Input: part model. Units: mm. Frame: model coordinates. Give positions to 0.01 mm unless a question says otherwise; leave off trailing zeros. Use CSV: the item, a comma, the result in double quotes. Start each with the question number.
Q1. Material intervals for line 1 along Z through (x, y) = (152, 2.9); line 2 along X through (y, z) = (3, -79.5); line 3 along X through (y, z) = (4.55, -16), sorted ascending.
Q2. Pin query (flat end, axial travel): pin 1 (1.5 mm diameter, centred on y = 2.5, z = -39, fed in from -X); pin 2 (2.5 mm diameter, centred on x = 96, z = -79.5, fed in from -Y); pin 3 (2 mm diameter, centred on y = 0.5, z = 15, fed in from +X); pin 4 (2 mm diameter, centred on x = 5, y = 3, fed in from -Z). Return the tip coordinate at first contact, or that it passes through.
Q3. Section A-A, the plane y = 3.25. State how many separate pieces and enclosed holes the cut face has, plus the area to 3 significant figures.
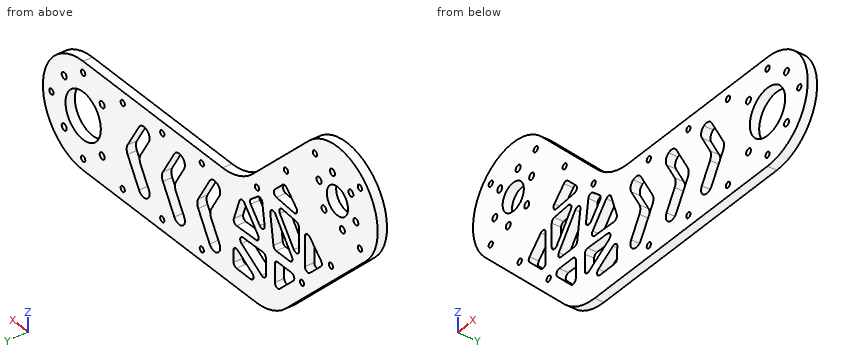
from build123d import *

# Parameters (mm, degrees)
SKETCH_1_R          = 28.5
EXTRUDE_1_DEPTH     = 5
FILLET_1_R          = 30
FILLET_2_R          = 30
CUT_EXTRUDE_1_DEPTH = 17
FILLET_3_R          = 5
FILLET_4_R          = 4
SKETCH_3_R          = 1.75
CUT_EXTRUDE_2_DEPTH = 22
SKETCH_4_R          = 1.75
CUT_EXTRUDE_3_DEPTH = 9
CUT_EXTRUDE_6_DEPTH = 10
FILLET_7_R          = 2
FILLET_8_R          = 2
SKETCH_8_R          = 1.5
CUT_EXTRUDE_7_DEPTH = 10
SKETCH_10_R         = 7.5
SKETCH_10_R_2       = 12.5
CUT_EXTRUDE_8_DEPTH = 10


with BuildPart() as part:
    # 草图1 → 凸台-拉伸1 (new body)
    with BuildSketch(Plane(origin=(0, 0, 0), x_dir=(1, 0, 0), z_dir=(0, 1, 0))):
        with BuildLine():
            Line((45.194913472, 85.5), (-20.152543264, 20.152543264))
            ThreePointArc((-20.152543264, 20.152543264), (10.906477822, 26.330566677), (28.5, 0))
            ThreePointArc((28.5, 0), (26.330566677, -10.906477822), (20.152543264, -20.152543264))
            Line((20.152543264, -20.152543264), (68.805086528, 28.5))
            Line((68.805086528, 28.5), (180, 28.5))
            ThreePointArc((180, 28.5), (151.5, 57), (180, 85.5))
            Line((180, 85.5), (45.194913472, 85.5))
        make_face()
        Circle(SKETCH_1_R)
        with Locations((180, 57)):
            Circle(SKETCH_1_R)
    extrude(amount=EXTRUDE_1_DEPTH)

    # 圆角1
    fillet_1_edges = [part.edges().sort_by_distance(p)[0] for p in [
        (68.805086528, 2.5, -28.5),
    ]]
    fillet(fillet_1_edges, radius=FILLET_1_R)

    # 圆角2
    fillet_2_edges = [part.edges().sort_by_distance(p)[0] for p in [
        (45.194913472, 2.5, -85.5),
    ]]
    fillet(fillet_2_edges, radius=FILLET_2_R)

    # 草图2 → 切除-拉伸1 (cut)
    with BuildSketch(Plane(origin=(0, 5, 0), x_dir=(1, 0, 0), z_dir=(0, 1, 0))):
        Polygon((150, 57), (138.452994616, 77), (131.524791386, 73), (140.762395693, 57), (131.524791386, 41), (138.452994616, 37), align=None)
        Polygon((106.524791386, 41), (115.762395693, 57), (106.524791386, 73), (113.452994616, 77), (125, 57), (113.452994616, 37), align=None)
        Polygon((81.524791386, 41), (90.762395693, 57), (81.524791386, 73), (88.452994616, 77), (100, 57), (88.452994616, 37), align=None)
    extrude(amount=-CUT_EXTRUDE_1_DEPTH, mode=Mode.SUBTRACT)

    # 圆角3
    fillet_3_edges = [part.edges().sort_by_distance(p)[0] for p in [
        (150, 2.5, -57),
        (140.762395693, 2.5, -57),
        (125, 2.5, -57),
        (115.762395693, 2.5, -57),
        (100, 2.5, -57),
        (90.762395693, 2.5, -57),
    ]]
    fillet(fillet_3_edges, radius=FILLET_3_R)

    # 圆角4
    fillet_4_edges = [part.edges().sort_by_distance(p)[0] for p in [
        (88.452994616, 2.5, -37),
        (81.524791386, 2.5, -41),
        (81.524791386, 2.5, -73),
        (106.524791386, 2.5, -73),
        (88.452994616, 2.5, -77),
        (113.452994616, 2.5, -77),
        (113.452994616, 2.5, -37),
        (106.524791386, 2.5, -41),
        (131.524791386, 2.5, -41),
        (138.452994616, 2.5, -37),
        (131.524791386, 2.5, -73),
        (138.452994616, 2.5, -77),
    ]]
    fillet(fillet_4_edges, radius=FILLET_4_R - 0.0001)  # a hair under: the kernel refuses the full size

    # 草图3 → 切除-拉伸2 (cut)
    with BuildSketch(Plane.XZ):
        with Locations(Location((193.435028843, -43.564971157, 0), (0, 0, 270))):
            Circle(SKETCH_3_R)
        with Locations(Location((193.435028843, -70.435028843, 0), (0, 0, 270))):
            Circle(SKETCH_3_R)
        with Locations(Location((166.564971157, -70.435028843, 0), (0, 0, 270))):
            Circle(SKETCH_3_R)
        with Locations(Location((166.564971157, -43.564971157, 0), (0, 0, 270))):
            Circle(SKETCH_3_R)
    extrude(amount=-CUT_EXTRUDE_2_DEPTH, mode=Mode.SUBTRACT)

    # 草图4 → 切除-拉伸3 (cut)
    with BuildSketch(Plane.XZ):
        with Locations(Location((3.494057109, 13.039998655, 0), (0, 0, 270))):
            Circle(SKETCH_4_R)
        with Locations(Location((-9.545941546, 9.545941546, 0), (0, 0, 270))):
            Circle(SKETCH_4_R)
        with Locations(Location((13.039998655, 3.494057109, 0), (0, 0, 270))):
            Circle(SKETCH_4_R)
        with Locations(Location((9.545941546, -9.545941546, 0), (0, 0, 270))):
            Circle(SKETCH_4_R)
        with Locations(Location((-3.494057109, -13.039998655, 0), (0, 0, 270))):
            Circle(SKETCH_4_R)
        with Locations(Location((-13.039998655, -3.494057109, 0), (0, 0, 270))):
            Circle(SKETCH_4_R)
    extrude(amount=-CUT_EXTRUDE_3_DEPTH, mode=Mode.SUBTRACT)

    # 草图7 → 切除-拉伸6 (cut)
    with BuildSketch(Plane(origin=(0, 5, 0), x_dir=(1, 0, 0), z_dir=(0, 1, 0))):
        Polygon((37.302376212, 11.879439437), (47.541331092, 22.118394317), (25.250183738, 23.931631911), align=None)
        Polygon((73.460547005, 75.506086264), (73.757768972, 63.62598632), (54.226268855, 75.506086264), align=None)
        Polygon((44.294954722, 72.402288525), (27.711693587, 55.81902739), (44.294954722, 55.81902739), align=None)
        Polygon((50.636885885, 71.015195544), (50.636885885, 56.423531637), (73.678593841, 57), align=None)
        Polygon((53.527673936, 52.761285689), (74.259925291, 53.279974973), (68.127983229, 35.438389149), align=None)
        Polygon((53.678821017, 27.188173586), (62.701661284, 34.792921342), (50.530965527, 49.233143064), align=None)
        Polygon((45.047320543, 50.522356459), (29.922245502, 50.522356459), (48.667218123, 25.171595633), align=None)
        Polygon((22.958665814, 52.076760267), (10.138217033, 39.256311486), (22.958665814, 26.435862705), align=None)
        Polygon((27.261857105, 47.74792215), (43.379167297, 25.950820384), (27.261857105, 27.261857105), align=None)
    extrude(amount=-CUT_EXTRUDE_6_DEPTH, mode=Mode.SUBTRACT)

    # 圆角7
    fillet_7_edges = [part.edges().sort_by_distance(p)[0] for p in [
        (44.294954722, 2.5, -72.402288525),
        (44.294954722, 2.5, -55.81902739),
        (27.711693587, 2.5, -55.81902739),
        (50.636885885, 2.5, -71.015195544),
        (73.678593841, 2.5, -57),
        (50.636885885, 2.5, -56.423531637),
        (68.127983229, 2.5, -35.438389149),
        (53.527673936, 2.5, -52.761285689),
        (74.259925291, 2.5, -53.279974973),
        (53.678821017, 2.5, -27.188173586),
        (50.530965527, 2.5, -49.233143064),
        (62.701661284, 2.5, -34.792921342),
        (45.047320543, 2.5, -50.522356459),
        (48.667218123, 2.5, -25.171595633),
        (29.922245502, 2.5, -50.522356459),
        (54.226268855, 2.5, -75.506086264),
        (73.460547005, 2.5, -75.506086264),
        (73.757768972, 2.5, -63.62598632),
    ]]
    fillet(fillet_7_edges, radius=FILLET_7_R)

    # 圆角8
    fillet_8_edges = [part.edges().sort_by_distance(p)[0] for p in [
        (37.302376212, 2.5, -11.879439437),
        (25.250183738, 2.5, -23.931631911),
        (47.541331092, 2.5, -22.118394317),
        (22.958665814, 2.5, -52.076760267),
        (22.958665814, 2.5, -26.435862705),
        (10.138217033, 2.5, -39.256311486),
        (27.261857105, 2.5, -27.261857105),
        (27.261857105, 2.5, -47.74792215),
        (43.379167297, 2.5, -25.950820384),
    ]]
    fillet(fillet_8_edges, radius=FILLET_8_R)

    # 草图8 → 切除-拉伸7 (cut)
    with BuildSketch(Plane(origin=(0, 5, 0), x_dir=(1, 0, 0), z_dir=(0, 1, 0))):
        with Locations(Location((-15.909902577, -15.909902577, 0), (0, 0, 270))):
            Circle(SKETCH_8_R)
        with Locations(Location((-15.909902577, 15.909902577, 0), (0, 0, 270))):
            Circle(SKETCH_8_R)
        with Locations(Location((15.909902577, -15.909902577, 0), (0, 0, 270))):
            Circle(SKETCH_8_R)
        with Locations(Location((4.596194078, 36.415999231, 0), (0, 0, 270))):
            Circle(SKETCH_8_R)
        with Locations(Location((25.102290732, 56.922095886, 0), (0, 0, 270))):
            Circle(SKETCH_8_R)
        with Locations(Location((36.415999231, 4.596194078, 0), (0, 0, 270))):
            Circle(SKETCH_8_R)
        with Locations(Location((56.922095886, 25.102290732, 0), (0, 0, 270))):
            Circle(SKETCH_8_R)
        with Locations(Location((180, 79.5, 0), (0, 0, 270))):
            Circle(SKETCH_8_R)
        with Locations(Location((180, 34.5, 0), (0, 0, 270))):
            Circle(SKETCH_8_R)
        with Locations(Location((152, 79.5, 0), (0, 0, 270))):
            Circle(SKETCH_8_R)
        with Locations(Location((124, 79.5, 0), (0, 0, 270))):
            Circle(SKETCH_8_R)
        with Locations(Location((96, 79.5, 0), (0, 0, 270))):
            Circle(SKETCH_8_R)
        with Locations(Location((152, 34.5, 0), (0, 0, 270))):
            Circle(SKETCH_8_R)
        with Locations(Location((124, 34.5, 0), (0, 0, 270))):
            Circle(SKETCH_8_R)
        with Locations(Location((96, 34.5, 0), (0, 0, 270))):
            Circle(SKETCH_8_R)
        with Locations(Location((202.5, 57, 0), (0, 0, 270))):
            Circle(SKETCH_8_R)
    extrude(amount=-CUT_EXTRUDE_7_DEPTH, mode=Mode.SUBTRACT)

    # 草图10 → 切除-拉伸8 (cut)
    with BuildSketch(Plane(origin=(0, 5, 0), x_dir=(1, 0, 0), z_dir=(0, 1, 0))):
        with Locations(Location((0, 0, 0), (0, 0, 270))):
            Circle(SKETCH_10_R)
        with Locations(Location((180, 57, 0), (0, 0, 270))):
            Circle(SKETCH_10_R_2)
    extrude(amount=-CUT_EXTRUDE_8_DEPTH, mode=Mode.SUBTRACT)


solid = part.part
A:
1,line 1,"-85.5 to -81, -78 to -36, -33 to -28.5"
1,line 2,"39.62 to 94.5, 97.5 to 122.5, 125.5 to 150.5, 153.5 to 178.5, 181.5 to 197.49"
1,line 3,"-23.58 to -17.41, -14.41 to 33.18, 41.42 to 56.31"
2,pin 1,"x = -2.06"
2,pin 2,"through"
2,pin 3,"x = 26.31"
2,pin 4,"z = -46.31"
3,separate pieces,"1"
3,enclosed holes,"40"
3,area,"11,100 mm^2"
